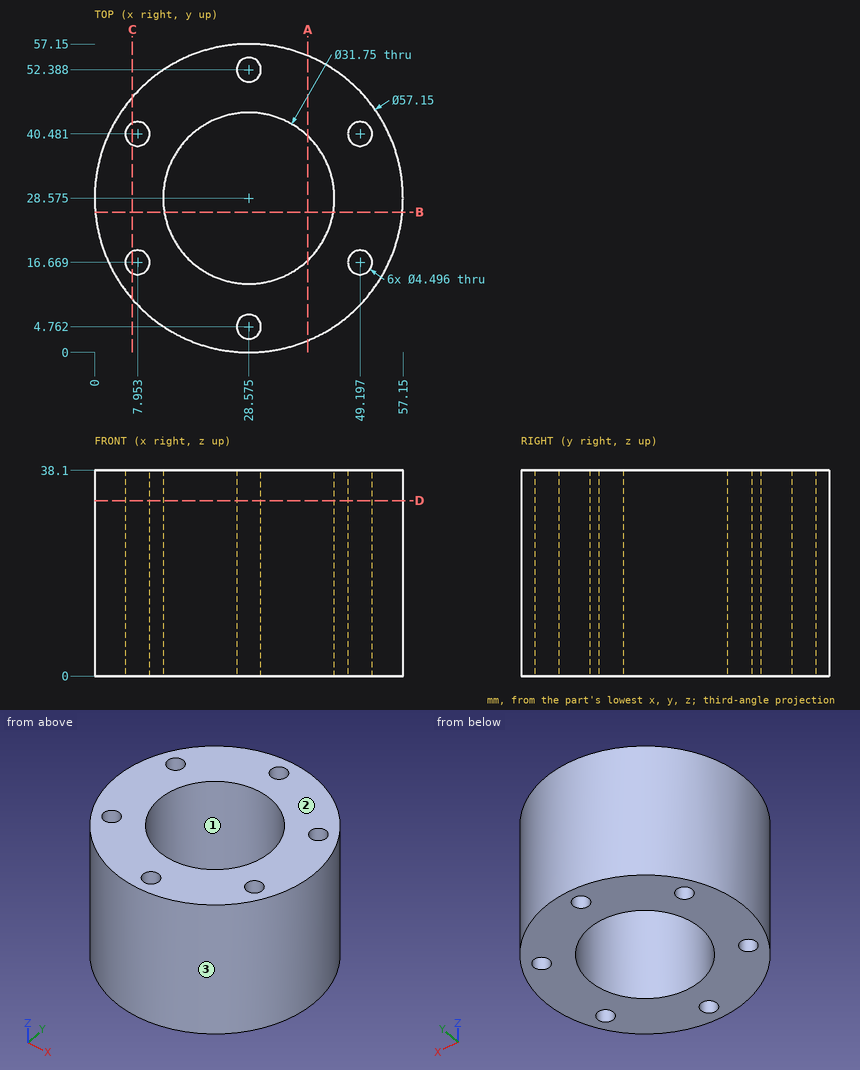
Print and shaded views of the part. All mm, measured from the part's lowest x, y and z. Round coordinates to 2 decimals unless told otherwise and drop trailing zeros. Order: outer loops, then holes, each group sorted by start corner. A loop starts at its lowest first (then second) coordinate and runs counter-clockwise, first axis right, second up. Notation, with made-up numbers: (24, 14.5) - (79, 14.5) arc R21 cw to (79, 26.5) - close; hole circle Ø1 at (-32, -18.5). An arc over 180 degrees is marked (long way). Use a Markdown table: item, result.
1) Saw through at D-D on z = 32.5. Give the number of separate pieces and of enclosed holes in the cut face, and give its area (3 significant figures).
Recorded:
| item | result |
|---|---|
| separate pieces | 1 |
| enclosed holes | 7 |
| area | 1,680 mm² |
2) Saw through at C-C on x = 7. Write the cut outline in (y, z) (1 decimal), and give its area (3 significant figures).
Recorded:
| item | result |
|---|---|
| outline | (9.8, 0) - (14.6, 0) - (14.6, 38.1) - (9.8, 38.1) - close; (18.7, 0) - (38.4, 0) - (38.4, 38.1) - (18.7, 38.1) - close; (42.5, 0) - (47.3, 0) - (47.3, 38.1) - (42.5, 38.1) - close |
| area | 1,120 mm² |
3) Saw through at A-A on x = 39.5. Write the cut outline in (y, z), and give its area (3 significant figures).
Recorded:
| item | result |
|---|---|
| outline | (2.17, 0) - (17.06, 0) - (17.06, 38.1) - (2.17, 38.1) - close; (40.09, 0) - (54.98, 0) - (54.98, 38.1) - (40.09, 38.1) - close |
| area | 1,130 mm² |
4) Flat gauge pins, fed straight in: pin 1 Ø4 at (x, y) = (49.2, 40.48) entering from +Z; pin 2 Ø12 at (y, z) = (49, 31) entering from +X; pin 3 Ø2 at (x, z) = (48, 14) entering from +Y (1 decimal); pin 4 Ø2 at (y, z) = (20, 10.5) entering from +X. Where does each tip first touch, or does it go through?
Recorded:
| item | result |
|---|---|
| pin 1 | passes through |
| pin 2 | stops at x = 53.24 |
| pin 3 | stops at y = 50.4 |
| pin 4 | stops at x = 56.13 |
5) Wall check: L1, parallel to Y at x = 49.5, z = 7 (1 decimal); L2, parallel to X at y = 29, z = 14.5 (1 decimal); L3, parallel to Y at x = 51, z = 24 (1 decimal). Give the ranges that are in metal, low to high.
Recorded:
| item | result |
|---|---|
| L1 | y = 9.1 to 14.4, 18.9 to 38.3, 42.7 to 48 |
| L2 | x = 0 to 12.7, 44.4 to 57.1 |
| L3 | y = 10.9 to 15.3, 18 to 39.1, 41.8 to 46.3 |
6) Pull direction X, two halves, no side cores. Call the marked faces 1, 2 and 3: pulls with the +X half, pulls with the -X half, needs draft (parallel to the pull), parting line crosses it, or undercut.
Recorded:
| item | result |
|---|---|
| face 1 | undercut |
| face 2 | needs draft |
| face 3 | parting line crosses it |
7) Saw through at B-B on y = 26. Write the cut outline in (x, z), and give its area (3 significant figures).
Recorded:
| item | result |
|---|---|
| outline | (0.12, 0) - (12.91, 0) - (12.91, 38.1) - (0.12, 38.1) - close; (44.24, 0) - (57.03, 0) - (57.03, 38.1) - (44.24, 38.1) - close |
| area | 975 mm² |
